Autodesk Inventor part; units mm, degrees
ref_plane "YZ Plane" through (0, 0, 0) normal (1, 0, 0) x (0, 1, 0)
ref_plane "XZ Plane" through (0, 0, 0) normal (0, 1, 0) x (-1, 0, 0)
ref_plane "XY Plane" through (0, 0, 0) normal (0, 0, 1) x (1, 0, 0)
sketch "Sketch1" plane through (0, 0, 0) normal (0, 1, 0) x (-1, 0, 0)
  line L0 (0, 0) -> (10, 0)
  line L1 (0, 0) -> (20, 0)
  line L2 (20, 0) -> (20, -20)
  line L3 (20, -20) -> (0, -20)
  line L4 (0, -10) -> (0, 0)
  line L5 (10, -10) -> (10, -20)
  line L6 (10, -10) -> (0, -10)
  dimension "d3" = 20
  dimension "d4" = 20
extrude "Extrusion1" add sketch "Sketch1" along normal blind 7.5
sketch "Sketch2" plane through (-10, 0, -10) normal (1, 0, 0) x (0, 0, -1)
  line L0 (0, 0) -> (10, 0)
  line L1 (10, 0) -> (10, 7.5)
  line L2 (0, 7.5) -> (10, 7.5)
  line L3 (0, 0) -> (0, 7.5)
  line L4 (-10, 0) -> (0, 0)
  line L5 (0, 0) -> (0, 7.5)
  line L6 (-10, 7.5) -> (0, 7.5)
  line L7 (-10, 0) -> (-10, 7.5)
  line L8 (10, 0) -> (10, 7.5)
  line L9 (10, 4.5) -> (-10, 4.5)
  point P0 (0, 4.5)
  dimension "d18" = 4.5
extrude "Extrusion2" cut sketch "Sketch2" against normal blind 5.3 contours L3 L9 L1 L0
sketch "Sketch3" plane through (0, 7.5, -10) normal (0, 0, -1) x (-1, 0, 0)
  line L0 (0, -7.5) -> (15.3, -7.5)
  line L1 (15.3, -7.5) -> (15.3, -3)
  line L2 (10, -3) -> (15.3, -3)
  line L3 (10, -3) -> (10, 0)
  line L4 (0, 0) -> (10, 0)
  line L5 (0, -7.5) -> (0, 0)
  line L6 (10, -3) -> (0, -3)
  line L7 (0, -7.5) -> (0, 0)
extrude "Extrusion3" cut sketch "Sketch3" against normal blind 5.3 contours L5 L6 L2 L1 L0
sketch "Sketch4" plane through (0, 0, 0) normal (0, -1, 0) x (1, 0, 0)
  line L0 (-15.3, -20) -> (-15.3, -4.7)
  line L1 (-15.3, -4.7) -> (0, -4.7)
  line L2 (0, 0) -> (0, -4.7)
  line L3 (-20, 0) -> (0, 0)
  line L4 (-20, -20) -> (-20, 0)
  line L5 (-15.3, -20) -> (-20, -20)
  line L6 (0, 0) -> (0, -10)
  circle A0 centre (-10.33, -2.5) radius 2
  circle A1 centre (-17.5, -9.67) radius 2
  dimension "d11" = 4
  dimension "d12" = 4
  dimension "d16" = 9.67
  dimension "d17" = 9.67
extrude "Extrusion4" add sketch "Sketch4" along normal blind 4 contours A0 | A1
fillet "Fillet1" radius 2 1 edges at (-20, 3.75, 0)
sketch "Sketch5" plane through (0, 7.5, 0) normal (0, 1, 0) x (1, 0, 0)
  arc A0 (-20, 2) -> (-18, 0) centre (-18, 2) ccw
  line L0 (-18, 0) -> (0, 0)
  line L1 (0, 0) -> (0, 10)
  line L2 (0, 10) -> (-10, 10)
  line L3 (-10, 10) -> (-10, 20)
  line L4 (-10, 20) -> (-20, 20)
  line L5 (-20, 20) -> (-20, 2)
  line L6 (2.5, 22.5) -> (-22.5, 22.5)
  line L7 (-22.5, 22.5) -> (-22.5, -2.5)
  line L8 (-22.5, -2.5) -> (2.5, -2.5)
  line L9 (2.5, -2.5) -> (2.5, 22.5)
  line L10 (2.5, 22.5) -> (-22.5, -2.5) construction
  line L11 (-22.5, 22.5) -> (2.5, -2.5) construction
  line L12 (-15.3, 20) -> (-20, 20)
  line L13 (-20, 20) -> (-22.5, 20)
  line L14 (0, 0) -> (0, -2.5)
  dimension "d19" = 25
  dimension "d20" = 25
extrude "Extrusion5" add sketch "Sketch5" against normal blind 7.5 contours A0 L0 L14 L8 L7 L13 L5
fillet "Fillet2" radius 5 1 edges at (-22.5, 3.75, 2.5)
properties part number "PresasPlaca_3DPrint"
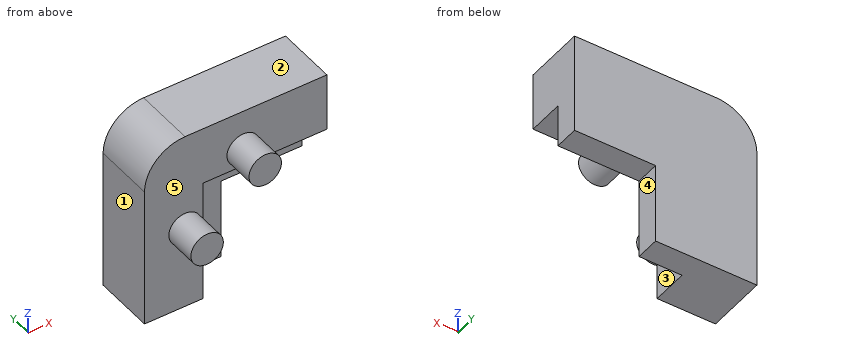
The listing builds one solid part. Answer for the finished solid, in the listing's coordinates (mm). Face numbers are marked on the shaded views. A direction names the side the tool comes from. Give positions to 0.01 mm unless a question says otherwise; leave off trailing zeros. Write each loop counter-clockwise with the first axis right and the second up, starting at its lowest first coordinate (ties: lowest second). Pieces come first, ordered by that corner, then holes. Notation, with made-up numbers: (22, 35.25) -> (26, 35.25) arc R4 cw to (26, 39.25) -> close; hole circle Ø1 at (30, 25.5). An arc over 180 degrees is marked (long way). Use one line per item in the form item = value.
1) Section C-C on y = -2.25 is taken. Write down the section's boundary in (x, z), plus the area to 3 significant figures.
Result:
outline = circle Ø4 at (-17.5, -9.67); circle Ø4 at (-10.33, -2.5)
area = 25.1 mm²
2) Straight lines are drawn through the part: probe 1 along X at (y, z) = (-1, -9.5); probe 2 along Z at (x, y) = (-9, 0.75); probe 3 along X at (y, z) = (0.75, -12.25). For each, find the intervals that lie inside material, in ascending order.
Result:
probe_1 = -19.49 to -15.51
probe_2 = -4.7 to 2.5
probe_3 = -22.5 to -15.3
3) Section B-B on y = 6.5 is taken. Write down the section's boundary in (x, z).
Result:
outline = (-22.5, -20) -> (-10, -20) -> (-10, -10) -> (0, -10) -> (0, 2.5) -> (-17.5, 2.5) arc R5 ccw to (-22.5, -2.5) -> close
4) Section A-A on x = -10.33 is taken. Write down the section's boundary in (y, z), plus the area to 3 significant figures.
Result:
outline = (-4, -4.5) -> (0, -4.5) -> (0, -4.7) -> (4.5, -4.7) -> (4.5, -20) -> (7.5, -20) -> (7.5, 2.5) -> (0, 2.5) -> (0, -0.5) -> (-4, -0.5) -> close
area = 116 mm²
5) Each of these flat-tipped pins is pushed along its axis until it touches: P1, Ø2.5, axis at y = 6, z = -13, coming from the +X side; P2, Ø2, axis at x = -12.5, y = 2, coming from the -Z side; P3, Ø2.5, axis at x = -6, y = 5.5, coming from the -Z side. Where does it stop, or does it pass through?
Result:
P1 = -10
P2 = -4.7
P3 = -10
6) A tool of negligible diameter and unlimited length cuts with its end or side. For the marked faces 1, 2, 3, 4 and 5, from which of +Z, -Z, +X, -X, +Y, -Y can it reach the whole face along a straight path? Write none if from no direction.
Result:
face_1 = +Z, -Z, -X, +Y, -Y
face_2 = +Z, +X, -X, +Y, -Y
face_3 = -Z, +X, -Y
face_4 = -Z, +X, +Y, -Y
face_5 = -Y
7) Section D-D on z = -16 is taken. Write down the section's boundary in (x, y).
Result:
outline = (-22.5, 0) -> (-15.3, 0) -> (-15.3, 4.5) -> (-10, 4.5) -> (-10, 7.5) -> (-22.5, 7.5) -> close
